```python
from build123d import *

# Parameters (mm, degrees)
BLANKSKE_W          = 25
BLANKSKE_H          = 7.3
BLANK_DEPTH         = 4
TOOTHCUTSIM_DEPTH   = 27.349383294
TEETHCUTS_COUNT     = 17
TEETHCUTS_PITCH     = 1.570796325
SKETCH4_W           = 25
SKETCH4_H           = 1.13
BOSS_EXTRUDE1_DEPTH = 2
BOSS_EXTRUDE2_DEPTH = 1
CUT_EXTRUDE1_DEPTH  = 27.519615382


with BuildPart() as part:
    # BlankSke → Blank (new body)
    with BuildSketch(Plane.XY):
        with Locations((12.5, 3.65)):
            Rectangle(BLANKSKE_W, BLANKSKE_H)
    extrude(amount=-BLANK_DEPTH)

    # TooCutSkeSim → ToothCutSim (cut, through all)
    with BuildSketch(Plane.XY):
        Polygon((0.222217685, 6.175), (-0.222217685, 6.175), (-0.640929042, 7.3254), (0.640929042, 7.3254), align=None)
    toothcutsim = extrude(amount=-TOOTHCUTSIM_DEPTH, mode=Mode.SUBTRACT)

    # TeethCuts: ToothCutSim ×17
    with Locations(*[(i * TEETHCUTS_PITCH, 0, 0) for i in range(1, TEETHCUTS_COUNT)]):
        add(toothcutsim, mode=Mode.SUBTRACT)

    # Sketch4 → Boss-Extrude1 (add)
    with BuildSketch(Plane.XZ):
        with Locations((12.5, -3.435)):
            Rectangle(SKETCH4_W, SKETCH4_H)
    extrude(amount=BOSS_EXTRUDE1_DEPTH)

    # Sketch7 → Boss-Extrude2 (add)
    with BuildSketch(Plane.XY):
        Polygon((25, 6.175), (24.910523515, 6.175), (24.501057002, 7.3), (24.193629073, 7.3), (23.78416256, 6.175), (23.33972719, 6.175), (22.930260677, 7.3), (22.622832748, 7.3), (22.213366235, 6.175), (21.768930865, 6.175), (21.359464352, 7.3), (21.052036423, 7.3), (20.64256991, 6.175), (20.19813454, 6.175), (19.788668027, 7.3), (19.481240098, 7.3), (19.071773585, 6.175), (18.627338215, 6.175), (18.217871702, 7.3), (17.910443773, 7.3), (17.50097726, 6.175), (17.05654189, 6.175), (16.647075377, 7.3), (16.339647448, 7.3), (15.930180935, 6.175), (15.485745565, 6.175), (15.076279052, 7.3), (14.768851123, 7.3), (14.35938461, 6.175), (13.91494924, 6.175), (13.505482727, 7.3), (13.198054798, 7.3), (12.788588285, 6.175), (12.344152915, 6.175), (11.934686402, 7.3), (11.627258473, 7.3), (11.21779196, 6.175), (10.77335659, 6.175), (10.363890077, 7.3), (10.056462148, 7.3), (9.646995635, 6.175), (9.202560265, 6.175), (8.793093752, 7.3), (8.485665823, 7.3), (8.07619931, 6.175), (7.63176394, 6.175), (7.222297427, 7.3), (6.914869498, 7.3), (6.505402985, 6.175), (6.060967615, 6.175), (5.651501102, 7.3), (5.344073173, 7.3), (4.93460666, 6.175), (4.49017129, 6.175), (4.080704777, 7.3), (3.773276848, 7.3), (3.363810335, 6.175), (2.919374965, 6.175), (2.509908452, 7.3), (2.202480523, 7.3), (1.79301401, 6.175), (1.34857864, 6.175), (0.939112127, 7.3), (0.631684198, 7.3), (0.222217685, 6.175), (0, 6.175), (0, 0), (25, 0), align=None)
    extrude(amount=BOSS_EXTRUDE2_DEPTH)

    # Sketch1 → Cut-Extrude1 (cut, through all)
    with BuildSketch(Plane(origin=(0, 0, -4), x_dir=(-1, 0, 0), z_dir=(0, 0, -1))):
        with BuildLine():
            Line((-23, 1), (-23, 2))
            Line((-23, 2), (-24, 2))
            ThreePointArc((-24, 2), (-23.707106781, 1.292893219), (-23, 1))
        make_face()
        with BuildLine():
            Line((-24, 2), (-23, 2))
            Line((-23, 2), (-23, 3))
            ThreePointArc((-23, 3), (-23.707106781, 2.707106781), (-24, 2))
        make_face()
        with BuildLine():
            Line((-23, 3), (-23, 2))
            Line((-23, 2), (-23, 1))
            ThreePointArc((-23, 1), (-22.292893219, 1.292893219), (-22, 2))
            ThreePointArc((-22, 2), (-22.292893219, 2.707106781), (-23, 3))
        make_face()
        with BuildLine():
            ThreePointArc((-17, 2), (-18.5, 3.5), (-20, 2))
            Line((-20, 2), (-17, 2))
        make_face()
        with BuildLine():
            Line((-17, 2), (-20, 2))
            ThreePointArc((-20, 2), (-18.5, 0.5), (-17, 2))
        make_face()
        with BuildLine():
            ThreePointArc((-13, 2), (-14, 3), (-15, 2))
            Line((-15, 2), (-13, 2))
        make_face()
        with BuildLine():
            Line((-13, 2), (-15, 2))
            ThreePointArc((-15, 2), (-14, 1), (-13, 2))
        make_face()
        with BuildLine():
            ThreePointArc((-3, 2), (-4, 3), (-5, 2))
            Line((-5, 2), (-3, 2))
        make_face()
        with BuildLine():
            Line((-3, 2), (-5, 2))
            ThreePointArc((-5, 2), (-4, 1), (-3, 2))
        make_face()
    extrude(amount=-CUT_EXTRUDE1_DEPTH, mode=Mode.SUBTRACT)


solid = part.part
```
CAD build for the part. Positions are in the model's coordinates, mm. A direction names the side the tool comes from. Round coordinates to 2 decimals unless told otherwise and drop trailing zeros. Write each loop counter-clockwise with the first axis right and the second up, starting at its lowest first coordinate (ties: lowest second). Pieces come first, ordered by that corner, then holes. Notation, with made-up numbers: (69, -32) -> (81, -32) arc R17 cw to (81, -21) -> close; hole circle Ø5 at (52.25, -9.5). An arc over 180 degrees is marked (long way). Answer in a Markdown table with one row per item. Add a question column.
Item 1: Which spindle directions (+Z, -Z, +X, -X, +Y, -Y) get a long thin tool onto all of the face, cutting with end or side? Do faces 4 (the face through (12, -1, -2.87)), 5 (the face through (12, 4, 1)). Say none if no direction does.
Item 2: Saw through at A-A, the plane y = 1.75. Write the cut outline in (x, z).
Item 3: Mould opens along Y. For faces 1 (the face through (0, 3, -2)), 2 (the face through (3, 2, -2)), 3 (the face through (12, 0, -1)) say: pulls with the +Y half, pulls with the -Y half, needs draft (parallel to the pull), parting line crosses it, or undercut.
Item 4: Drop a flat-ended pin along its axis: pin 1 Ø2.5 at (x, y) = (14, 2) entering from +Z. Give the stop position or say it passes through.
Item 5: Saw through at B-B, the plane z = -3.4. Count the separate pieces of the cut face and the enclosed holes in it, then the cut area to 3 significant figures.
Item 6: Drill centre lines: line 1 (X direction, y = 2, z = -0.05); line 2 (Y direction, x = 14, z = -1.2) (3 decimals); line 3 (Z direction, x = 4.75, y = -0.75). Where is each one in solid material? Low to high. Write a range as from..to.
Findings below:
| question | item | result |
|---|---|---|
| 1 | face 4 | +Z, +X, -X, -Y |
| 1 | face 5 | +Z, +X, -X, +Y, -Y |
| 2 | outline | (0, -4) -> (3.03, -4) -> (3.03, 1) -> (0, 1) -> close; (4.97, -4) -> (13.03, -4) -> (13.03, 1) -> (4.97, 1) -> close; (14.97, -4) -> (17.02, -4) -> (17.02, 1) -> (14.97, 1) -> close; (19.98, -4) -> (22.03, -4) -> (22.03, 1) -> (19.98, 1) -> close; (23.97, -4) -> (25, -4) -> (25, 1) -> (23.97, 1) -> close |
| 3 | face 1 | needs draft |
| 3 | face 2 | undercut |
| 3 | face 3 | pulls with the -Y half |
| 4 | pin 1 | stops at z = 1 |
| 5 | separate pieces | 1 |
| 5 | enclosed holes | 4 |
| 5 | area | 201 mm^2 |
| 6 | line 1 | x = 0..3, 5..13, 15..17, 20..22, 24..25 |
| 6 | line 2 | y = 0..1, 3..6.175 |
| 6 | line 3 | z = -4..-2.87 |
